Geometry check sheet. Reference: the model listing, model coordinates, mm. A direction names the side the tool comes from. Give positions to 0.01 mm unless a question says otherwise; leave off trailing zeros. Write each loop counter-clockwise with the first axis right and the second up, starting at its lowest first coordinate (ties: lowest second). Pieces come first, ordered by that corner, then holes. Notation, with made-up numbers: (69.25, 57.25) - (114.25, 57.25) arc R15 cw to (114.25, 69.25) - close; hole circle Ø2 at (88, -1). An arc over 180 degrees is marked (long way). One line per question, with ' | ' between items. Start each with the question number.
Q1. Section check A-A on x = 20.5. Record the boundary of the cut face in (y, z), and give its area (3 significant figures).
Q2. Section check C-C on y = -14.5. Record the boundary of the cut face in (x, z).
Q3. Set-up check for faces 1 (the face through (-82.53, -9.01, 185.44)), 2 (the face through (1, -5, 17.78)): record each of +Z, -Z, +X, -X, +Y, -Y from which the full face is reachable in a straight line by a thin tool's end or side.
Q4. Section check B-B on z = 117. Record the boundary of the cut face in (x, y).
Q5. Gauge pin test, flat ends, axial feed: P1, Ø1.5, axis at y = -5.5, z = 190, coming from the -X side; P2, Ø19.5, axis at x = -26, z = 13, coming from the +Y side; P3, Ø3, axis at y = -11.5, z = 309, coming from the -X side; P4, Ø2, axis at x = 45, y = -8.5, coming from the -Z side. Record the tip position at first contact, or that the pin passes through.
Q6. Thickness scan on L1, parallel to Z at x = -63, y = -9.25; L2, parallel to X at y = -1, z = 50; L3, parallel to X at y = -16.25, z = 175. Record the ranges inside material, lowest first. Write a range as [from, to].
```python
from build123d import *

# Parameters (mm, degrees)
F0_W     = 177.8
F0_H     = 365.76
F1_DEPTH = 17.78
F2_W     = 177.8
F2_H     = 17.78
F3_DEPTH = 10.16
F5_DEPTH = 365.761


with BuildPart() as f1:
    # F0 (on Front) → F1 (new body)
    with BuildSketch(Plane.XZ):
        with Locations((0, 182.88)):
            Rectangle(F0_W, F0_H)
    extrude(amount=F1_DEPTH)

    # F2 (on face) → F3 (cut)
    with BuildSketch(Plane(origin=(0, 0, 0), x_dir=(-1, 0, 0), z_dir=(0, 1, 0))):
        with Locations((0, 8.89)):
            Rectangle(F2_W, F2_H)
    extrude(amount=-F3_DEPTH, mode=Mode.SUBTRACT)

    # F4 (on face) → F5 (cut, through all)
    with BuildSketch(Plane.XY.offset(365.76)):
        Polygon((-88.9, 0), (-88.9, -17.78), (-75.982074, 0), align=None)
        Polygon((75.982074, 0), (88.9, -17.78), (88.9, 0), align=None)
    extrude(amount=-F5_DEPTH, mode=Mode.SUBTRACT)


solid = f1.part
```
Working result:
1) outline: (-17.78, 0) - (-10.16, 0) - (-10.16, 17.78) - (0, 17.78) - (0, 365.76) - (-17.78, 365.76) - close | area: 6,320 mm2
2) outline: (-86.52, 0) - (86.52, 0) - (86.52, 365.76) - (-86.52, 365.76) - close
3) face 1: +Z, -Z, -X, +Y | face 2: -Z, +X, -X, +Y
4) outline: (-88.9, -17.78) - (88.9, -17.78) - (75.98, 0) - (-75.98, 0) - close
5) P1: stops at x = -80.52 | P2: stops at y = 0 | P3: stops at x = -85.43 | P4: stops at z = 17.78
6) L1: z = [17.78, 365.76] | L2: x = [-76.71, 76.71] | L3: x = [-87.79, 87.79]
